```python
from build123d import *

# Parameters (mm, degrees)
SKETCH_1_W        = 30
SKETCH_1_H        = 60
EXTRUDE_1_DEPTH   = 2
CHAMFER_1_SIZE    = 2
HOLE_WIZARD_M61_D = 6.6


with BuildPart() as part:
    # Эскиз1 → Бобышка-Вытянуть1 (new body)
    with BuildSketch(Plane.XY):
        Rectangle(SKETCH_1_W, SKETCH_1_H)
    extrude(amount=EXTRUDE_1_DEPTH)

    # Фаска1
    chamfer_1_edges = [part.edges().sort_by_distance(p)[0] for p in [
        (15, -30, 1),
        (-15, -30, 1),
        (-15, 30, 1),
        (15, 30, 1),
    ]]
    chamfer(chamfer_1_edges, length=CHAMFER_1_SIZE)

    # Отверстие с зазором M61 (through all)
    with Locations(Plane.XY.offset(2)):
        with Locations((0, -45), (0, 45), (0, 15), (0, -15)):
            Hole(HOLE_WIZARD_M61_D / 2)


solid = part.part
```
Input: part model. Units: mm. Frame: model coordinates. Round coordinates to 2 decimals unless told otherwise and drop trailing zeros. Loops run counter-clockwise (first coordinate to the right, second up) from the corner with the lowest first, then second, coordinate; pieces in that order, holes last. Notation, with made-up numbers: (65.5, 55) -> (113.5, 55) arc R14 ccw to (113.5, 77) -> close; hole circle Ø2 at (-11, 26.5). An arc over 180 degrees is marked (long way). Use one line per item in the form item = value. Start each with the question number.
Item 1: Section query A-A on z = 0.6. Return the cut outline in (x, y), then the cut area to 3 significant figures.
Item 2: Material intervals for L1, parallel to Y at x = 0, z = 1.6; L2, parallel to Y at x = -2.75, z = 0.25; L3, parallel to X at y = 12, z = 0.95, sorted ascending. Write a range as from..to.
Item 3: Mould query, pull axis Y, two halves, no side actions, for faces 1 (the face through (-15, 0, 1)), 2 (the face through (0, -30, 1)), 3 (the face through (2.43, 17.23, 0.99)). Classes: pulls with the +Y half, pulls with the -Y half, needs draft (parallel to the pull), parting line crosses it, or undercut.
Item 4: Contact query for a flat-ended pin moving along its axis: pin 1 Ø8.5 at (x, y) = (0, 15) entering from -Z. Output: stop coordinate, or through.
Item 5: Section query C-C on y = 14. Return the cut outline in (x, z).
Item 6: Section query B-B on x = 0. Return the cut outline in (y, z).
Item 7: Section query D-D on y = -15. Return the cut outline in (x, z).
Ans:
q1.outline = (-15, -28) -> (-13, -30) -> (13, -30) -> (15, -28) -> (15, 28) -> (13, 30) -> (-13, 30) -> (-15, 28) -> close; hole circle Ø6.6 at (0, -15); hole circle Ø6.6 at (0, 15)
q1.area = 1,720 mm^2
q2.L1 = -30..-18.3, -11.7..11.7, 18.3..30
q2.L2 = -30..-16.82, -13.18..13.18, 16.82..30
q2.L3 = -15..-1.37, 1.37..15
q3.face_1 = needs draft
q3.face_2 = pulls with the -Y half
q3.face_3 = undercut
q4.pin_1 = 0
q5.outline = (-15, 0) -> (-3.14, 0) -> (-3.14, 2) -> (-15, 2) -> close; (3.14, 0) -> (15, 0) -> (15, 2) -> (3.14, 2) -> close
q6.outline = (-30, 0) -> (-18.3, 0) -> (-18.3, 2) -> (-30, 2) -> close; (-11.7, 0) -> (11.7, 0) -> (11.7, 2) -> (-11.7, 2) -> close; (18.3, 0) -> (30, 0) -> (30, 2) -> (18.3, 2) -> close
q7.outline = (-15, 0) -> (-3.3, 0) -> (-3.3, 2) -> (-15, 2) -> close; (3.3, 0) -> (15, 0) -> (15, 2) -> (3.3, 2) -> close
